Input: part model. Units: mm. Frame: model coordinates. Face numbers are marked on the shaded views. A direction names the side the tool comes from. Coordinates: 2 decimals unless noted, no trailing zeros. Order: outer loops, then holes, each group sorted by start corner. A loop starts at its lowest first (then second) coordinate and runs counter-clockwise, first axis right, second up. Notation, with made-up numbers: (-19.5, -34.5) - (-9.5, -34.5) arc R4 cw to (-9.5, -28.5) - close; hole circle Ø11 at (64.25, 79). An arc over 180 degrees is marked (long way). One line per question, with ' | ' between items.
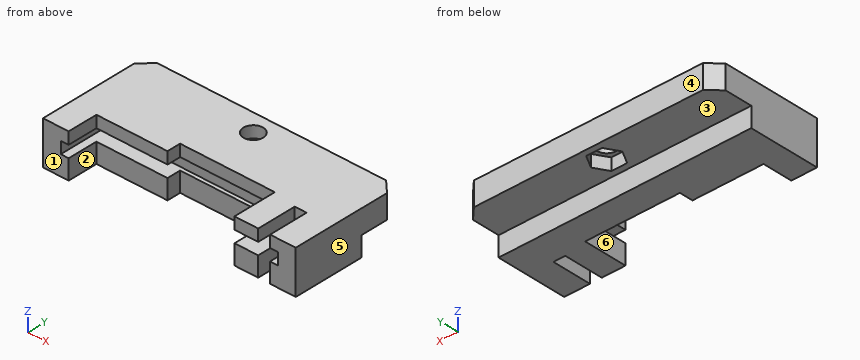
from build123d import *

# Parameters (mm, degrees)
SKETCH_R        = 2.5
PAD_DEPTH       = 11
SKETCH001_W     = 72.573656
SKETCH001_H     = 10
POCKET_DEPTH    = 5
POCKET001_DEPTH = 3.05
SKETCH003_W     = 55
SKETCH003_H     = 3
POCKET002_DEPTH = 12


with BuildPart() as part:
    # Sketch → Pad (new body)
    with BuildSketch(Plane.XY):
        Polygon((-32, -28), (-32, -3), (-29, 0), (29, 0), (32, -3), (32, -28), (25.5, -28), (25.5, -18), (22.5, -18), (22.5, -28), (16.5, -28), (16.5, -16.95), (-7.5, -16.95), (-7.5, -20.4), (-25.5, -20.4), (-25.5, -28), align=None)
        with Locations((0, -5)):
            Circle(SKETCH_R, mode=Mode.SUBTRACT)
    extrude(amount=PAD_DEPTH)

    # Sketch001 (on Face18 of Pad) → Pocket (cut)
    with BuildSketch(Plane(origin=(0, 0, 0), x_dir=(1, 0, 0), z_dir=(0, 0, -1))):
        with Locations((0, 5)):
            Rectangle(SKETCH001_W, SKETCH001_H)
    extrude(amount=-POCKET_DEPTH, mode=Mode.SUBTRACT)

    # Sketch002 (on Face4 of Pocket) → Pocket001 (cut)
    with BuildSketch(Plane(origin=(0, 0, 5), x_dir=(1, 0, 0), z_dir=(0, 0, -1))):
        Polygon((3.983717, 5), (1.991858, 8.45), (-1.991858, 8.45), (-3.983717, 5), (-1.991858, 1.55), (1.991858, 1.55), align=None)
    extrude(amount=-POCKET001_DEPTH, mode=Mode.SUBTRACT)

    # Sketch003 (on Face17 of Pocket001) → Pocket002 (cut)
    with BuildSketch(Plane.XZ.offset(28)):
        with Locations((0, 6.5)):
            Rectangle(SKETCH003_W, SKETCH003_H)
    extrude(amount=-POCKET002_DEPTH, mode=Mode.SUBTRACT)


solid = part.part
Item 1: Section A-A on x = 0. Return the cut outline in (y, z).
Data:
outline: (-16.95, 0) - (-10, 0) - (-10, 5) - (-8.45, 5) - (-8.45, 8.05) - (-7.5, 8.05) - (-7.5, 11) - (-16.95, 11) - (-16.95, 8) - (-16, 8) - (-16, 5) - (-16.95, 5) - close; (-2.5, 8.05) - (-1.55, 8.05) - (-1.55, 5) - (0, 5) - (0, 11) - (-2.5, 11) - close
Item 2: Section D-D on x = -13. Return the cut outline in (y, z), and give its area (3 significant figures).
Data:
outline: (-20.4, 0) - (-10, 0) - (-10, 5) - (0, 5) - (0, 11) - (-20.4, 11) - (-20.4, 8) - (-16, 8) - (-16, 5) - (-20.4, 5) - close | area: 161 mm^2
Item 3: Section C-C on y = -26. Return the cut outline in (x, z), and give its area (3 significant figures).
Data:
outline: (-32, 0) - (-25.5, 0) - (-25.5, 5) - (-27.5, 5) - (-27.5, 8) - (-25.5, 8) - (-25.5, 11) - (-32, 11) - close; (16.5, 0) - (22.5, 0) - (22.5, 5) - (16.5, 5) - close; (16.5, 8) - (22.5, 8) - (22.5, 11) - (16.5, 11) - close; (25.5, 0) - (32, 0) - (32, 11) - (25.5, 11) - (25.5, 8) - (27.5, 8) - (27.5, 5) - (25.5, 5) - close | area: 179 mm^2
Item 4: Section B-B on z = 5.75. Return the cut outline in (x, y).
Data:
outline: (-32, -28) - (-27.5, -28) - (-27.5, -16) - (27.5, -16) - (27.5, -28) - (32, -28) - (32, -3) - (29, 0) - (-29, 0) - (-32, -3) - close; hole (-3.98, -5) - (-1.99, -8.45) - (1.99, -8.45) - (3.98, -5) - (1.99, -1.55) - (-1.99, -1.55) - close
Item 5: Ray query, line 1 (X direction, y = -20.5, z = 9.25); line 2 (X direction, y = -19.25, z = 3.25); line 3 (X direction, y = -5, z = 8.7). Return the intervals inside material, ascending.
Data:
line 1: -32 to -25.5, 16.5 to 22.5, 25.5 to 32 | line 2: -32 to -7.5, 16.5 to 22.5, 25.5 to 32 | line 3: -32 to -2.5, 2.5 to 32
Item 6: Access query for the marked faces 1, 2 and 3. Directions: +Z, -Z, +X, -X, +Y, -Y. A direction counts if a zero-diameter tool reaches every point of the face in a straight line with its end or side. Return the directions, or none.
Data:
face 1: +Z, -Z, +X, -X, -Y | face 2: +Z, -Z, -Y | face 3: -Z, +X, -X, +Y
Item 7: Draft query along X for the marked faces 4, 5 and 6. Return one class per face: released by +X, released by -X, zero draft, split by the parting line, or undercut.
Data:
face 4: zero draft | face 5: released by +X | face 6: undercut
Item 8: Contact query for flat-ended pins moving along their axis: P1, Ø6, axis at x = 12, z = 2, coming from the -Y side; P2, Ø3, axis at x = 15.5, z = 2, coming from the +Y side; P3, Ø2.5, axis at x = 24, z = 9, coming from the -Y side; P4, Ø4.5, axis at x = 0, y = -5, coming from the +Z side. Output: stop coordinate, or through.
Data:
P1: y = -16.95 | P2: y = -10 | P3: y = -18 | P4: through
